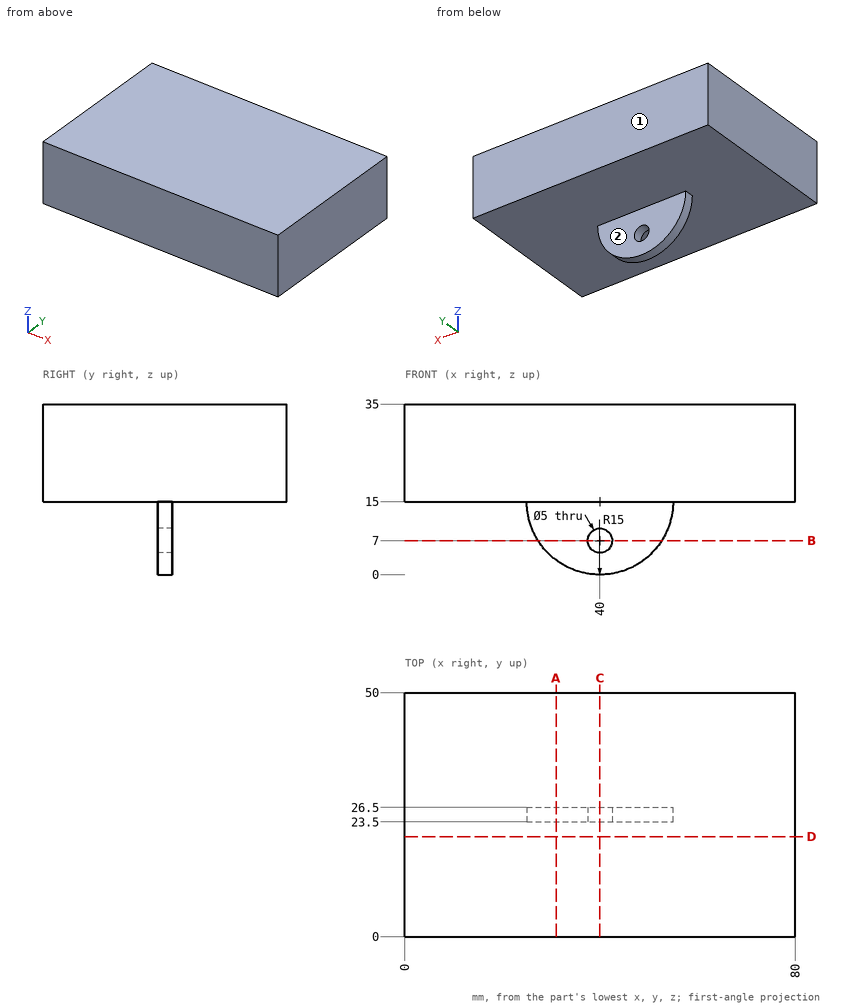
Could you check a few things on this drawing? It's one solid part, dimensions in mm from its lowest x, y, z. A direction names the side the tool comes from. Round coordinates to 2 decimals unless told otherwise and drop trailing zeros. Order: outer loops, then holes, each group sorted by start corner. A loop starts at its lowest first (then second) coordinate and runs counter-clockwise, first axis right, second up. Notation, with made-up numbers: M 23,30 L 39,30 A21 cw 39,35 Z; hole C 82.25,65 d2. An arc over 180 degrees is marked long. Use a Markdown table: item, result.
1) Imagine slicing it at D-D (y = 20.5). List the corners of the cut face in (x, z) for me, then the cut area to 3 significant figures.
Geometry says:
| item | result |
|---|---|
| outline | M 0,15 L 80,15 L 80,35 L 0,35 Z |
| area | 1,600 mm² |
2) If I drill on line 1 along Z through (x, y) = (21, 25.5); line 2 along X through (y, z) = (26, 8.5); line 3 along X through (y, z) = (24.2, 7), over which ranges is the centre line in solid material (lowest first)?
Geometry says:
| item | result |
|---|---|
| line 1 | z = 15 to 35 |
| line 2 | x = 26.48 to 38, 42 to 53.52 |
| line 3 | x = 27.31 to 37.5, 42.5 to 52.69 |
3) Imagine slicing it at B-B (z = 7). List the corners of the cut face in (x, y) for me.
Geometry says:
| item | result |
|---|---|
| outline | M 27.31,23.5 L 37.5,23.5 L 37.5,26.5 L 27.31,26.5 Z; M 42.5,23.5 L 52.69,23.5 L 52.69,26.5 L 42.5,26.5 Z |
4) On a 3-axis mill with a long thin cutter (end or side, diameter ignored), from which of +Z, -Z, +X, -X, +Y, -Y can I reach the whole of each face in a straight line? I mean the marked faces 1 and 2. Say none if no direction works.
Geometry says:
| item | result |
|---|---|
| face 1 | +Z, -Z, +X, -X, +Y |
| face 2 | -Z, +X, -X, +Y |
5) Imagine slicing it at A-A (x = 31). List the corners of the cut face in (y, z) for me.
Geometry says:
| item | result |
|---|---|
| outline | M 0,15 L 23.5,15 L 23.5,3 L 26.5,3 L 26.5,15 L 50,15 L 50,35 L 0,35 Z |
6) I'm going to push flat-ended pins straight in: P1, Ø6.5, axis at x = 40, z = 7, coming from the +Y side; P2, Ø8, axis at y = 24, z = 17.5, coming from the -X side; P3, Ø25, axis at x = 58.5, y = 22, coming from the -Z side; P4, Ø7.5, axis at x = 43.5, z = 10, coming from the -Y side. Where does each tip first touch, or does it pass through?
Geometry says:
| item | result |
|---|---|
| P1 | stops at y = 26.5 |
| P2 | stops at x = 0 |
| P3 | stops at z = 1.29 |
| P4 | stops at y = 23.5 |
7) Imagine slicing it at C-C (x = 40). List the corners of the cut face in (y, z) for me.
Geometry says:
| item | result |
|---|---|
| outline | M 0,15 L 23.5,15 L 23.5,9.5 L 26.5,9.5 L 26.5,15 L 50,15 L 50,35 L 0,35 Z; M 23.5,0 L 26.5,0 L 26.5,4.5 L 23.5,4.5 Z |
